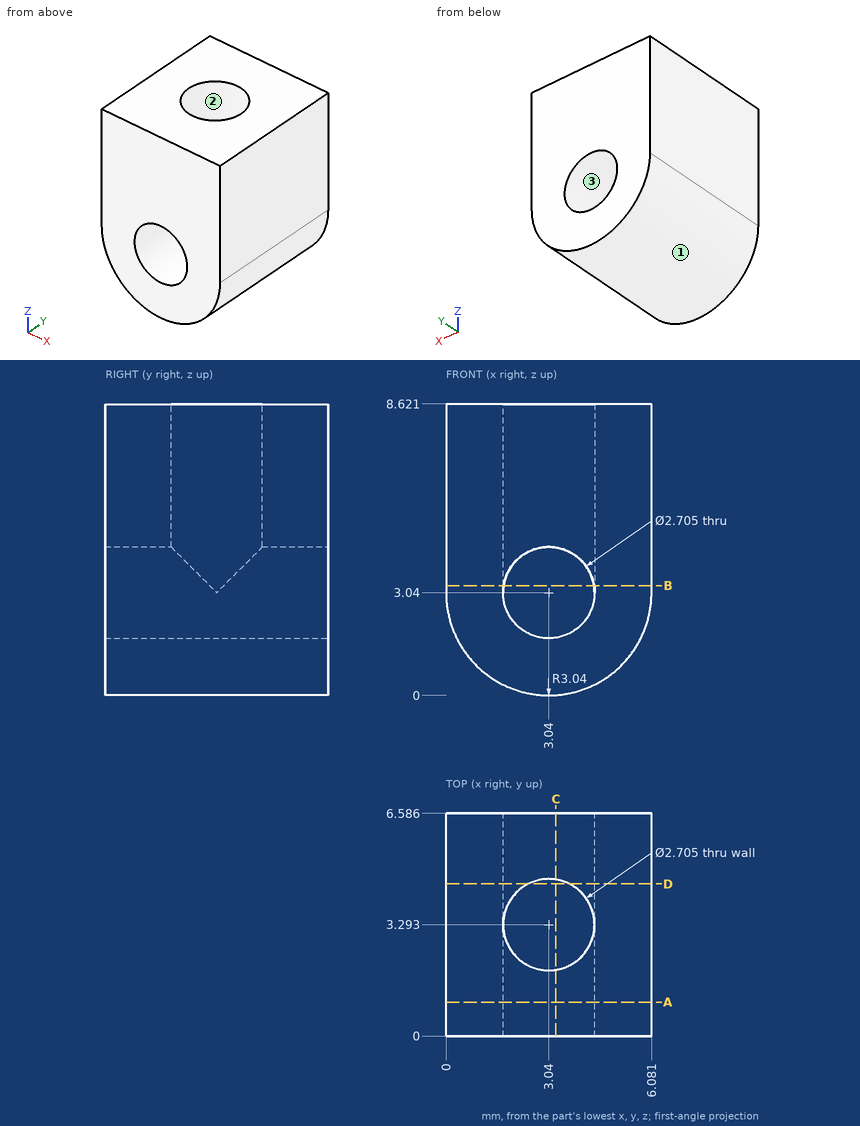
Design review of the part shown in the three views and the two pictorial views. Dimensions are in mm from the part's minimum x, y and z. Give positions to 0.01 mm unless a question says otherwise; leave off trailing zeros. Loops run counter-clockwise (first coordinate to the right, second up) from the corner with the lowest first, then second, coordinate; pieces in that order, holes last. Notation, with made-up numbers: (83.25, -4) - (113.25, -4) arc R28 cw to (113.25, 15) - close; hole circle Ø2 at (6.5, 69). An arc over 180 degrees is marked (long way). Write item = value, one per line.
1) Take a section at A-A on y = 1. State the section outline as (x, z) points (1 decimal), and give its area (3 significant figures).
Result sheet:
outline = (0, 3) arc R3 ccw to (6.1, 3) - (6.1, 8.6) - (0, 8.6) - close; hole circle Ø2.7 at (3, 3)
area = 42.7 mm2
2) To check wall thickness, follow line 1 (X direction, y = 6.5, z = 3.75); line 2 (X direction, y = 4.25, z = 7) (1 decimal); line 3 (Z direction, x = 4, y = 5) (1 decimal). State the ranges of each line that lie inside material, in increasing order.
Result sheet:
line_1 = 0 to 1.89, 4.19 to 6.08
line_2 = 0 to 2.1, 4 to 6.1
line_3 = 0.2 to 2.1, 4 to 8.6
3) Take a section at C-C on x = 3.25. State the section outline as (y, z) points, and give its area (3 significant figures).
Result sheet:
outline = (0, 0.01) - (6.59, 0.01) - (6.59, 1.7) - (0, 1.7) - close; (0, 4.38) - (1.96, 4.38) - (1.96, 8.62) - (0, 8.62) - close; (4.63, 4.38) - (6.59, 4.38) - (6.59, 8.62) - (4.63, 8.62) - close
area = 27.8 mm2
4) Take a section at B-B on z = 3.25. State the section outline as (x, y) points (1 decimal).
Result sheet:
outline = (0, 0) - (1.7, 0) - (1.7, 3.1) arc R1.4 cw to (1.7, 3.5) - (1.7, 6.6) - (0, 6.6) - close; (4.4, 0) - (6.1, 0) - (6.1, 6.6) - (4.4, 6.6) - (4.4, 3.5) arc R1.4 cw to (4.4, 3.1) - close
5) Take a section at D-D on y = 4.5. State the section outline as (x, z) points (1 decimal).
Result sheet:
outline = (0, 3) arc R3 ccw to (6.1, 3) - (6.1, 8.6) - (3.7, 8.6) - (3.7, 4.2) arc R1.4 cw (long way) to (2.4, 4.2) - (2.4, 8.6) - (0, 8.6) - close
6) Draft analysis for pull direction Z (two halves, no side actions). For the marked faces 1, 2 and 3, state which applies: +Z half, -Z half, draft (parallel to the pull), parting line (faces both ways), or undercut.
Result sheet:
face_1 = -Z half
face_2 = draft
face_3 = undercut
